```python
from build123d import *

# Parameters (mm, degrees)
SM_BASE_FLANGE_1_DEPTH = 100
SM_EDGE_FLANGE_1_DEPTH = 97.6


# Sheet-metal steps are written as plain solids
with BuildPart() as part:
    # Sketch 1 → 基体-法兰1 (new body)
    with BuildSketch(Plane(origin=(0, 0, 0), x_dir=(0, 0, -1), z_dir=(1, 0, 0))):
        with BuildLine():
            Line((0, 35), (0, 1.2))
            ThreePointArc((0, 1.2), (0.351471863, 0.351471863), (1.2, 0))
            Line((1.2, 0), (98.8, 0))
            ThreePointArc((98.8, 0), (99.648528137, 0.351471863), (100, 1.2))
            Line((100, 1.2), (100, 35))
            Line((100, 35), (99, 35))
            Line((99, 35), (99, 1.2))
            ThreePointArc((99, 1.2), (98.941421356, 1.058578644), (98.8, 1))
            Line((98.8, 1), (1.2, 1))
            ThreePointArc((1.2, 1), (1.058578644, 1.058578644), (1, 1.2))
            Line((1, 1.2), (1, 35))
            Line((1, 35), (0, 35))
        make_face()
    extrude(amount=SM_BASE_FLANGE_1_DEPTH)

    # 边线-法兰1 section (across the edge) → 边线-法兰1 (add)
    with BuildSketch(Plane(origin=(100.2, 1, -1.2), x_dir=(-1, 0, 0), z_dir=(0, 0, -1))):
        with BuildLine():
            Line((-1, 0.2), (-1, 34))
            Line((-1, 34), (0, 34))
            Line((0, 34), (0, 0.2))
            ThreePointArc((0, 0.2), (0.058578644, 0.058578644), (0.2, 0))
            Line((0.2, 0), (0.2, -1))
            ThreePointArc((0.2, -1), (-0.648528137, -0.648528137), (-1, 0.2))
        make_face()
    extrude(amount=SM_EDGE_FLANGE_1_DEPTH)


solid = part.part
```
Input: part model. Units: mm. Frame: model coordinates. A direction names the side the tool comes from. Coordinates: 2 decimals unless noted, no trailing zeros. Loops run counter-clockwise (first coordinate to the right, second up) from the corner with the lowest first, then second, coordinate; pieces in that order, holes last. Notation, with made-up numbers: (41, -37.75) -> (91, -37.75) arc R21 cw to (91, 0.25) -> close; hole circle Ø9 at (50, 75). An arc over 180 degrees is marked (long way). Use a Markdown table: item, result.
1) Cut plane B-B (x = 23). Return the cut outline in (y, z).
Results found:
| item | result |
|---|---|
| outline | (0, -98.8) arc R1.2 ccw to (1.2, -100) -> (35, -100) -> (35, -99) -> (1.2, -99) arc R0.2 cw to (1, -98.8) -> (1, -1.2) arc R0.2 cw to (1.2, -1) -> (35, -1) -> (35, 0) -> (1.2, 0) arc R1.2 ccw to (0, -1.2) -> close |
2) Access query for faces 4 (the flat face through (101.2, 18, -49)), 5 (the flat face through (49, 1, -51)), 6 (the flat face through (49, 18, -99)). Directions: +Z, -Z, +X, -X, +Y, -Y. A direction counts if a zero-diameter tool reaches every point of the face in a straight line with its end or side. Return the directions, or none.
Results found:
| item | result |
|---|---|
| face 4 | +Z, -Z, +X, +Y, -Y |
| face 5 | -X, +Y |
| face 6 | +X, -X, +Y |
3) Material intervals for line 1 along Z through (x, y) = (65.5, 19); line 2 along X through (y, z) = (8.5, -15); line 3 along Y through (x, z) = (10.5, -26.5), sorted ascending. Write a range as from..to.
Results found:
| item | result |
|---|---|
| line 1 | z = -100..-99, -1..0 |
| line 2 | x = 100.2..101.2 |
| line 3 | y = 0..1 |
4) Pull-direction query (Z, two-part tool) for faces 1 (the flat face through (49, 18, -1)), 2 (the flat face through (100.2, 18, -49)), 3 (the flat face through (49, 18, -100)); classes: released by +Z, released by -Z, zero draft, split by the parting line, or undercut.
Results found:
| item | result |
|---|---|
| face 1 | undercut |
| face 2 | zero draft |
| face 3 | released by -Z |
5) Cut plane A-A (y = 16). Return the cut outline in (x, z), then the cut area to 3 significant figures.
Results found:
| item | result |
|---|---|
| outline | (0, -100) -> (100, -100) -> (100, -99) -> (0, -99) -> close; (0, -1) -> (100, -1) -> (100, 0) -> (0, 0) -> close; (100.2, -98.8) -> (101.2, -98.8) -> (101.2, -1.2) -> (100.2, -1.2) -> close |
| area | 298 mm2 |
6) Contact query for flat-ended pins moving along their axis: pin 1 (6 mm diameter, centred on y = 18, z = -61.5, fed in from -X); pin 2 (1.3 mm diameter, centred on x = 101, y = 20, fed in from +Z); pin 3 (1 mm diameter, centred on y = 25, z = -0.5, fed in from +X). Output: stop coordinate, or through.
Results found:
| item | result |
|---|---|
| pin 1 | stops at x = 100.2 |
| pin 2 | stops at z = -1.2 |
| pin 3 | stops at x = 100 |
7) Cut plane C-C (z = -54). Return the cut outline in (x, y).
Results found:
| item | result |
|---|---|
| outline | (0, 0) -> (100, 0) arc R1.2 ccw to (101.2, 1.2) -> (101.2, 35) -> (100.2, 35) -> (100.2, 1.2) arc R0.2 cw to (100, 1) -> (0, 1) -> close |
